Answer from the drawing. Dimensions are ordinates in mm from the lowest x, y and z of the part. A direction names the side the tool comes from. Give positions to 0.01 mm unless a question says otherwise; leave off trailing zeros. Write each loop counter-clockwise with the first axis right and the second up, starting at its lowest first coordinate (ties: lowest second). Pieces come first, ordered by that corner, then holes. Notation, with made-up numbers: M 53,28.5 L 62,28.5 A13 cw 62,51.5 Z; hole C 46,-32 d5. An arc over 180 degrees is marked long. Answer as a JSON object with one key per item and string values.
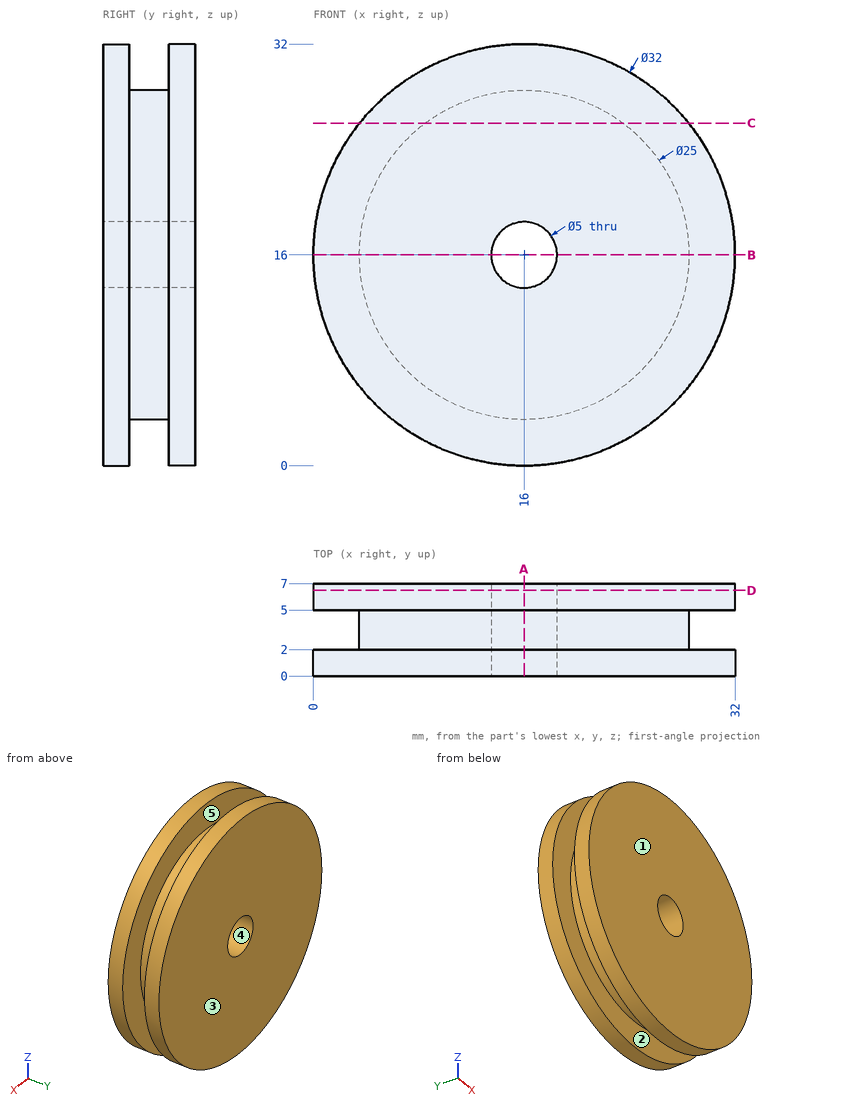
1. A cutting plane is placed at C-C, the plane z = 26. Give the vertices of the cut face in (x, y).
Verdict:
{"outline": "M 3.51,0 L 28.49,0 L 28.49,2 L 23.5,2 L 23.5,5 L 28.49,5 L 28.49,7 L 3.51,7 L 3.51,5 L 8.5,5 L 8.5,2 L 3.51,2 Z"}
2. A cutting plane is placed at B-B, the plane z = 16. Give the vertices of the cut face in (x, y), plus the area to 3 significant figures.
Verdict:
{"outline": "M 0,0 L 13.5,0 L 13.5,7 L 0,7 L 0,5 L 3.5,5 L 3.5,2 L 0,2 Z; M 18.5,0 L 32,0 L 32,2 L 28.5,2 L 28.5,5 L 32,5 L 32,7 L 18.5,7 Z", "area": "168 mm2"}
3. The mould has two halves that part along Y. Classify the marked faces 3, 4 and 5: released by +Y, released by -Y, zero draft, split by the parting line, or undercut.
Verdict:
{"face 3": "released by +Y", "face 4": "zero draft", "face 5": "undercut"}
4. A cutting plane is placed at A-A, the plane x = 16. Give the vertices of the cut face in (y, z), plus the area to 3 significant figures.
Verdict:
{"outline": "M 0,0 L 2,0 L 2,3.5 L 5,3.5 L 5,0 L 7,0 L 7,13.5 L 0,13.5 Z; M 0,18.5 L 7,18.5 L 7,32 L 5,32 L 5,28.5 L 2,28.5 L 2,32 L 0,32 Z", "area": "168 mm2"}
5. A flat-ended cylindrical pin translates along its axis: pin 1 (3 mm diameter, centred on x = 10.5, y = 4, fed in from +Z). Find the tip coordinate at first contact, or state that the pin passes through.
Verdict:
{"pin 1": "stops at z = 31.39"}
6. For the marked faces 1 and 2, determine the directions among +Z, -Z, +X, -X, +Y, -Y from which every point of the face is accessible in a straight line to the end or side of a thin tool.
Verdict:
{"face 1": "+Z, -Z, +X, -X, -Y", "face 2": "none"}
7. Consider line 1 along Y through (x, z) = (29.5, 16.5); line 2 along Z through (x, y) = (16, 2.25); line 3 along Z through (x, y) = (17, 3.25). Determine where each line is inside the solid, lowest interval first.
Verdict:
{"line 1": "y = 0 to 2, 5 to 7", "line 2": "z = 3.5 to 13.5, 18.5 to 28.5", "line 3": "z = 3.54 to 13.71, 18.29 to 28.46"}
8. A cutting plane is placed at D-D, the plane y = 6.5. Give the vertices of the cut face in (x, z).
Verdict:
{"outline": "C 16,16 d32; hole C 16,16 d5"}
